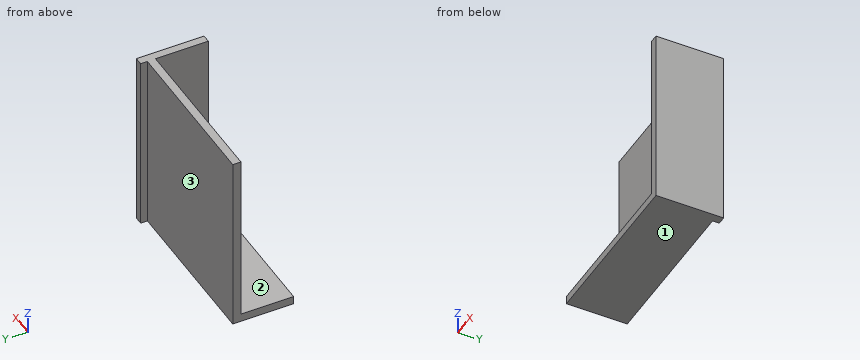
from build123d import *

# Parameters (mm, degrees)
SKETCH_2_W      = 240
SKETCH_2_H      = 270
EXTRUDE_1_DEPTH = 12
SKETCH_3_W      = 270
SKETCH_3_H      = 100
EXTRUDE_2_DEPTH = 12
SKETCH_4_W      = 12
SKETCH_4_H      = 78
EXTRUDE_3_DEPTH = 240


with BuildPart() as part:
    # 草图2 → 凸台-拉伸1 (new body)
    with BuildSketch(Plane(origin=(0, 0, 0), x_dir=(1, 0, 0), z_dir=(0, 1, 0))):
        with Locations((120, 135)):
            Rectangle(SKETCH_2_W, SKETCH_2_H)
    extrude(amount=EXTRUDE_1_DEPTH)

    # 草图3 → 凸台-拉伸2 (add)
    with BuildSketch(Plane(origin=(240, 0, 0), x_dir=(0, 0, -1), z_dir=(1, 0, 0))):
        with Locations((135, -28)):
            Rectangle(SKETCH_3_W, SKETCH_3_H)
    extrude(amount=EXTRUDE_2_DEPTH)

    # 草图4 → 凸台-拉伸3 (add)
    with BuildSketch(Plane.ZY.offset(-240)):
        with Locations((-264, -39)):
            Rectangle(SKETCH_4_W, SKETCH_4_H)
    extrude(amount=EXTRUDE_3_DEPTH)


solid = part.part
Verification items for the finished model (mm, model axes). Face numbers are marked on the shaded views. A direction names the side the tool comes from. Round coordinates to 2 decimals unless told otherwise and drop trailing zeros. Loops run counter-clockwise (first coordinate to the right, second up) from the corner with the lowest first, then second, coordinate; pieces in that order, holes last. Notation, with made-up numbers: M -12,89 L 40,89 A20 ccw 40,126 Z; hole C 56,53 d5. An arc over 180 degrees is marked long. Write each question's results on one line, items separated by ' | '.
1) Gauge pin test, flat ends, axial feed: P1, Ø5, axis at y = 15, z = -193.5, coming from the -X side; P2, Ø1, axis at x = 59, z = -239, coming from the -Y side. Record the tip position at first contact, or that the pin passes through.
Checks:
P1: stops at x = 240 | P2: stops at y = 0
2) Section check C-C on x = 32. Record the boundary of the cut face in (y, z), then the cut area to 3 significant figures.
Checks:
outline: M -78,-270 L 12,-270 L 12,0 L 0,0 L 0,-258 L -78,-258 Z | area: 4,180 mm2
3) Scan lines: L1, parallel to X at y = -21, z = -47; L2, parallel to Z at x = 24, y = -32; L3, parallel to Y at x = 156.5, z = -51.5. Record each from-to range of solid material in increasing order. Write a range as from..to.
Checks:
L1: x = 240..252 | L2: z = -270..-258 | L3: y = 0..12
4) Access from +Z, -Z, +X, -X, +Y, -Y to the whole of each face (thin tool, end or side, straight path). Record for the marked faces 1, 2 and 3.
Checks:
face 1: -Z, +X, -X, +Y, -Y | face 2: +Z, -X, -Y | face 3: +Z, -Z, -X, +Y
5) Section check A-A on y = -33.5. Record the boundary of the cut face in (x, z), then the cut area to 3 significant figures.
Checks:
outline: M 0,-270 L 252,-270 L 252,0 L 240,0 L 240,-258 L 0,-258 Z | area: 6,120 mm2
6) Section check B-B on z = -65. Record the boundary of the cut face in (x, y).
Checks:
outline: M 0,0 L 240,0 L 240,-78 L 252,-78 L 252,22 L 240,22 L 240,12 L 0,12 Z
